from build123d import *

# Parameters (mm, degrees)
EXTRUDE_1_DEPTH          = 30
EXTRUDE_START            = -30
EXTRUDE_2_DEPTH          = 30
EXTRUDE_3_DEPTH          = 30
EXTRUDE_START_2          = -2
SKETCH_9_W               = 5
SKETCH_9_H               = 46.18577558
EXTRUDE_6_DEPTH          = 22
FILLET_3_R               = 1
CUT_EXTRUDE_4_DEPTH      = 59.377928803
CUT_EXTRUDE_4_DEPTH_BACK = 59.377928803
SKETCH_10_R              = 2.1
CUT_EXTRUDE_5_DEPTH      = 3


with BuildPart() as part:
    # 草图1 → 凸台-拉伸1 (new body)
    with BuildSketch(Plane.XY):
        with BuildLine():
            Line((-23.903477417, 9.605041416), (-23.903477417, -9.460776308))
            ThreePointArc((-23.903477417, -9.460776308), (-22.605516257, -13.152827027), (-19.282718599, -15.22042404))
            Line((-19.282718599, -15.22042404), (-3.900036331, -18.636980321))
            ThreePointArc((-3.900036331, -18.636980321), (19.420354058, 0.072132554), (-3.900036331, 18.78124543))
            Line((-3.900036331, 18.78124543), (-19.282718599, 15.364689149))
            ThreePointArc((-19.282718599, 15.364689149), (-22.605516257, 13.297092136), (-23.903477417, 9.605041416))
        make_face()
        with BuildLine():
            ThreePointArc((-20.503477417, -9.460776308), (-19.953493875, -11.025204579), (-18.545528765, -11.901305008))
            Line((-18.545528765, -11.901305008), (-3.162846498, -15.317861289))
            ThreePointArc((-3.162846498, -15.317861289), (16.020354058, 0.072132554), (-3.162846498, 15.462126398))
            Line((-3.162846498, 15.462126398), (-18.545528765, 12.045570117))
            ThreePointArc((-18.545528765, 12.045570117), (-19.953493875, 11.169469687), (-20.503477417, 9.605041416))
            Line((-20.503477417, 9.605041416), (-20.503477417, -9.460776308))
        make_face(mode=Mode.SUBTRACT)
    extrude(amount=EXTRUDE_1_DEPTH)

    # 草图2 → 凸台-拉伸2 (add)
    with BuildSketch(Plane.XY.offset(30).offset(EXTRUDE_START)):
        with BuildLine():
            Line((0.255333714, -19.09288779), (-21.903477417, -19.09288779))
            ThreePointArc((-21.903477417, -19.09288779), (-23.31769098, -18.507101352), (-23.903477417, -17.09288779))
            Line((-23.903477417, -17.09288779), (-23.903477417, -9.460776308))
            Line((-23.903477417, -9.460776308), (-20.503477417, -9.460776308))
            ThreePointArc((-20.503477417, -9.460776308), (-19.953493875, -11.025204579), (-18.545528765, -11.901305008))
            Line((-18.545528765, -11.901305008), (-3.162846498, -15.317861289))
            ThreePointArc((-3.162846498, -15.317861289), (-1.464012153, -15.598850703), (0.255333714, -15.69288779))
            Line((0.255333714, -15.69288779), (0.255333714, -19.09288779))
        make_face()
    extrude_2 = extrude(amount=EXTRUDE_2_DEPTH)

    # 草图3 → 凸台-拉伸3 (add)
    with BuildSketch(Plane(origin=(0, 0, 0), x_dir=(-1, 0, 0), z_dir=(0, 0, -1))):
        with BuildLine():
            Line((21.903477417, -19.09288779), (21.903477417, -23.09288779))
            ThreePointArc((21.903477417, -23.09288779), (21.610584198, -23.799994571), (20.903477417, -24.09288779))
            Line((20.903477417, -24.09288779), (0, -24.09288779))
            ThreePointArc((0, -24.09288779), (-8.201928623, -22.653821067), (-15.42405585, -18.508531632))
            ThreePointArc((-15.42405585, -18.508531632), (-16.141619311, -17.062720423), (-15.557886921, -15.557886921))
            Line((-15.557886921, -15.557886921), (-13.642327271, -13.642327271))
            ThreePointArc((-13.642327271, -13.642327271), (-7.482369871, -17.678021056), (-0.255333714, -19.09288779))
            Line((-0.255333714, -19.09288779), (21.903477417, -19.09288779))
        make_face()
    extrude_3 = extrude(amount=-EXTRUDE_3_DEPTH)

    # 镜向1: 凸台-拉伸2, 凸台-拉伸3 across plane
    add(extrude_2.mirror(Plane.ZX))
    add(extrude_3.mirror(Plane.ZX))

    # 草图9 → 凸台-拉伸6 (add)
    with BuildSketch(Plane.ZY.offset(23.903477417).offset(EXTRUDE_START_2)):
        with Locations((2.5, 0)):
            Rectangle(SKETCH_9_W, SKETCH_9_H)
        with Locations((27.5, 0)):
            Rectangle(SKETCH_9_W, SKETCH_9_H)
    extrude(amount=EXTRUDE_6_DEPTH)

    # 圆角3
    fillet_3_edges = [part.edges().sort_by_distance(p)[0] for p in [
        (-43.903477417, 23.09288779, 27.5),
        (-43.903477417, -23.09288779, 27.5),
        (-43.903477417, 23.09288779, 2.5),
        (-43.903477417, -23.09288779, 2.5),
    ]]
    fillet(fillet_3_edges, radius=FILLET_3_R)

    # 草图10 → 切除-拉伸4 (cut, two sides: drawn at the far end of the back side and taken through both)
    with BuildSketch(Plane.XY.offset(30).offset(-CUT_EXTRUDE_4_DEPTH_BACK)):
        with Locations((-32.403477417, 10)):
            Circle(SKETCH_10_R)
        with Locations((-32.403477417, -10)):
            Circle(SKETCH_10_R)
    extrude(amount=CUT_EXTRUDE_4_DEPTH + CUT_EXTRUDE_4_DEPTH_BACK, mode=Mode.SUBTRACT)

    # 草图11 → 切除-拉伸5 (cut)
    with BuildSketch(Plane.XY.offset(30)):
        Polygon((-28.403477417, -10), (-30.403477417, -6.535898385), (-34.403477417, -6.535898385), (-36.403477417, -10), (-34.403477417, -13.464101615), (-30.403477417, -13.464101615), align=None)
        Polygon((-28.403477417, 10), (-30.403477417, 13.464101615), (-34.403477417, 13.464101615), (-36.403477417, 10), (-34.403477417, 6.535898385), (-30.403477417, 6.535898385), align=None)
    cut_extrude_5 = extrude(amount=-CUT_EXTRUDE_5_DEPTH, mode=Mode.SUBTRACT)

    # 镜向3: 切除-拉伸5 across plane
    add(cut_extrude_5.mirror(Plane.XY.offset(15)), mode=Mode.SUBTRACT)


solid = part.part
Can you work these out from the model? Positions are in its coordinate system, mm. A direction names the side the tool comes from. Round coordinates to 2 decimals unless told otherwise and drop trailing zeros. Loops run counter-clockwise (first coordinate to the right, second up) from the corner with the lowest first, then second, coordinate; pieces in that order, holes last. Notation, with made-up numbers: (55, 56) - (59, 56) arc R8 ccw to (59, 70) - close; hole circle Ø10 at (0.5, 38). An arc over 180 degrees is marked (long way). Answer in a Markdown table with one row per item. Add a question column.
Q1. For pin 1 Ø6 at (x, z) = (4, 23.5) entering from -Y; pin 2 Ø2.5 at (x, z) = (-33, 1) entering from -Y; pin 3 Ø10 at (x, z) = (11, 12) entering from +Y, each with a flat end and sliding along its axis, tell me the tip position at first contact or that it passes through.
Q2. We'd pull the mould along Y, two halves only. Please class faces 5 (the flat face through (-10.962, 13.586, 14.79)), 6 (the flat face through (-29.39, 11.71, 28.52)), 7 (the cylindrical face through (8.092, -22.693, 14.79)), 8 (the cylindrical face through (8.092, 22.693, 14.79)): pulls with the +Y half, pulls with the -Y half, needs draft (parallel to the pull), parting line crosses it, or undercut.
Q3. I want a section at A-A on z = 24.25. List the corners of the cut face in (x, y) for me.
Q4. Which directions (+Z, -Z, +X, -X, +Y, -Y) give clear straight access to the entire face, cutting with the end or side of a thin tool? Please do faces 1 (the flat face through (-29.42, 8.24, 1.48)), 2 (the flat face through (-32, 6.536, 29)), 3 (the cylindrical face through (15.88, -2.02, 14.79)), 4 (the flat face through (15, 15, 15)).
Q5. I want a section at C-C on y = 2.5. List the corners of the cut face in (x, z) for me, and give its area (3 significant figures).
Q6. I want a section at D-D on x = 7.5. List the corners of the cut face in (y, z) for me, and give its area (3 significant figures).
Q7. I want a section at B-B on x = -12.5. List the corners of the cut face in (y, z) for me.
Q8. I need wall thicknesses on L1, parallel to Z at x = -39.5, y = 11; L2, parallel to X at y = 10, z = 25.5; L3, parallel to X at y = -10, z = 26.5. Which ranges of each line are inside material? Lowest first, please.
A:
| question | item | result |
|---|---|---|
| 1 | pin 1 | y = -24.07 |
| 1 | pin 2 | y = -23.09 |
| 1 | pin 3 | y = 23.33 |
| 2 | face 5 | undercut |
| 2 | face 6 | undercut |
| 2 | face 7 | pulls with the -Y half |
| 2 | face 8 | pulls with the +Y half |
| 3 | outline | (-23.9, -17.09) arc R2 ccw to (-21.9, -19.09) - (-21.9, -23.09) arc R1 ccw to (-20.9, -24.09) - (0, -24.09) arc R24.09 ccw to (15.42, -18.51) arc R2 ccw to (15.56, -15.56) - (13.64, -13.64) arc R19.17 ccw to (13.72, 13.72) - (15.56, 15.56) arc R2 ccw to (15.42, 18.51) arc R24.09 ccw to (0, 24.09) - (-20.9, 24.09) arc R1 ccw to (-21.9, 23.09) - (-21.9, 19.09) arc R2 ccw to (-23.9, 17.09) - close; hole (-20.5, -9.46) arc R2.5 ccw to (-18.55, -11.9) - (-3.16, -15.32) arc R15.77 ccw (long way) to (0.26, 15.84) - (0.26, 15.69) arc R15.77 ccw to (-3.16, 15.32) - (-18.55, 11.9) arc R2.5 ccw to (-20.5, 9.46) - close |
| 4 | face 1 | -Z |
| 4 | face 2 | +Z |
| 4 | face 3 | +Z, -Z |
| 4 | face 4 | +Z, -Z, +X |
| 5 | outline | (-43.9, 0) - (-20.5, 0) - (-20.5, 30) - (-43.9, 30) - (-43.9, 25) - (-23.9, 25) - (-23.9, 5) - (-43.9, 5) - close; (15.83, 0) - (19.27, 0) - (19.27, 30) - (15.83, 30) - close |
| 5 | area | 405 mm^2 |
| 6 | outline | (-22.9, 0) - (-13.93, 0) - (-13.93, 30) - (-22.9, 30) - close; (14.07, 0) - (22.9, 0) - (22.9, 30) - (14.07, 30) - close |
| 6 | area | 534 mm^2 |
| 7 | outline | (-24.09, 0) - (-13.24, 0) - (-13.24, 30) - (-24.09, 30) - close; (13.24, 0) - (24.09, 0) - (24.09, 30) - (13.24, 30) - close |
| 8 | L1 | 0 to 5, 25 to 30 |
| 8 | L2 | -43.9 to -34.5, -30.3 to -20.44, 12.5 to 16.65 |
| 8 | L3 | -43.9 to -34.5, -30.3 to -20.44, 12.38 to 16.56 |
